```python
from build123d import *

# Parameters (mm, degrees)
F2_DEPTH  = 3
F1_R      = 2.5
F1_R_2    = 1.25
F3_DEPTH  = 10
F4_SIZE2  = 3
F4_SIZE   = 2
F5_R      = 2.99999
F7_W      = 10
F7_H      = 18
F8_DEPTH  = 4
F10_SIZE  = 1
F11_DEPTH = 33.6


# Not quite as in the source:
# - a fillet or chamfer is up to 0.001 mm smaller than in the source, because OpenCascade refuses the exact size


with BuildPart() as f2:
    # F0 (on Top) → F2 (new body)
    with BuildSketch(Plane.XY):
        with BuildLine():
            ThreePointArc((46, 18), (43.0710678119, 25.0710678119), (36, 28))
            Line((36, 28), (-36, 28))
            ThreePointArc((-36, 28), (-43.0710678119, 25.0710678119), (-46, 18))
            Line((-46, 18), (-46, -18))
            ThreePointArc((-46, -18), (-43.0710678119, -25.0710678119), (-36, -28))
            Line((-36, -28), (36, -28))
            ThreePointArc((36, -28), (43.0710678119, -25.0710678119), (46, -18))
            Line((46, -18), (46, 18))
        make_face()
    extrude(amount=F2_DEPTH)

    # F1 (on Top) → F3 (join)
    with BuildSketch(Plane.XY):
        with Locations((-29, 11.5)):
            Circle(F1_R)
        with Locations((-29, 11.5)):
            Circle(F1_R_2, mode=Mode.SUBTRACT)
        with Locations((29, 11.5)):
            Circle(F1_R)
        with Locations((29, 11.5)):
            Circle(F1_R_2, mode=Mode.SUBTRACT)
        with Locations((-29, -11.5)):
            Circle(F1_R)
        with Locations((-29, -11.5)):
            Circle(F1_R_2, mode=Mode.SUBTRACT)
        with Locations((29, -11.5)):
            Circle(F1_R)
        with Locations((29, -11.5)):
            Circle(F1_R_2, mode=Mode.SUBTRACT)
    extrude(amount=F3_DEPTH)

    # F4
    f4_edges = [f2.edges().sort_by_distance(p)[0] for p in [
        (-31.5, 11.5, 3),
        (26.5, 11.5, 3),
        (26.5, -11.5, 3),
        (-31.5, -11.5, 3),
    ]]
    chamfer(f4_edges, length=F4_SIZE, length2=F4_SIZE2)

    # F5 (radius 3 in the source; OpenCascade refuses exactly that, so slightly less here)
    f5_edges = [f2.edges().sort_by_distance(p)[0] for p in [
        (0, 28, 3),
    ]]
    fillet(f5_edges, radius=F5_R)

    # F7 (on offset) → F8 (join)
    with BuildSketch(Plane.YZ.offset(46)):
        with Locations((0, 9)):
            Rectangle(F7_W, F7_H)
    extrude(amount=-F8_DEPTH)

    # F9: F2 across plane


with BuildPart() as f2_1:
    add(f2.part)
    add(f2.part.mirror(Plane.YZ))

    # F10
    f10_edges = [f2_1.edges().sort_by_distance(p)[0] for p in [
        (-46, 0, 18),
        (46, 0, 18),
    ]]
    chamfer(f10_edges, length=F10_SIZE)

    # F11 (add): a face of the model
    f11_faces = [f2_1.faces().sort_by_distance(p)[0] for p in [
        (0, 0, 3),
    ]]
    extrude(f11_faces, amount=F11_DEPTH)


solid = f2_1.part
```
Here's how the part is built. I have some questions about the finished solid (model axes, mm). A direction names the side the tool comes from. Give positions to 0.01 mm unless a question says otherwise; leave off trailing zeros. Order: outer loops, then holes, each group sorted by start corner. A loop starts at its lowest first (then second) coordinate and runs counter-clockwise, first axis right, second up. Notation, with made-up numbers: M 36,1 L 74,1 A30 ccw 74,28 Z; hole C 14.5,67 d4. An arc over 180 degrees is marked long. Use a Markdown table: item, result. Add a question column.
1. For pin 1 Ø5 at (x, y) = (20.5, -5) entering from -Z; pin 2 Ø0.8 at (x, y) = (-29.5, 11) entering from +Z; pin 3 Ø0.9 at (x, z) = (-44.5, 8) entering from -Y; pin 4 Ø0.8 at (x, z) = (42.5, 29.5) entering from +Y, each with a flat end and sliding along its axis, tell me the tip position at first contact or that it passes through.
2. If we mould it in two halves opening along Y, with no side actions, what happens to faces 4 (the cylindrical face through (-24.708, 10.148, 19.565)), 5 (the flat face through (1, 0, 0)), 6 (the flat face through (-1, -25, 20)), 7 (the cylindrical face through (-0.5, 27.1, 2.14))? For each: +Y half, -Y half, draft (parallel to the pull), parting line (faces both ways), or undercut.
3. I need wall thicknesses on probe 1 along X at (y, z) = (-11.5, 27); probe 2 along Y at (x, z) = (29, 23); probe 3 along X at (y, z) = (-8.5, 30). Which ranges of each line are inside material? Lowest first, please. Write a range as from..to.
4. On a 3-axis mill with a long thin cutter (end or side, diameter ignored), from which of +Z, -Z, +X, -X, +Y, -Y can I reach the whole of each face in a straight line? I mean faces 1 (the flat face through (29, 12, 3)), 2 (the cylindrical face through (45.1, 11.59, 2.14)), 3 (the cylindrical face through (45.1, -11.41, 2.14)). Say none if no direction works.
5. Suppose I cut it at C-C (z = 15). List the corners of the cut face in (x, y) for me, and give its area (3 significant figures).
Results list:
| question | item | result |
|---|---|---|
| 1 | pin 1 | stops at z = 0 |
| 1 | pin 2 | stops at z = 3 |
| 1 | pin 3 | stops at y = -5 |
| 1 | pin 4 | stops at y = 21.43 |
| 2 | face 4 | undercut |
| 2 | face 5 | draft |
| 2 | face 6 | -Y half |
| 2 | face 7 | +Y half |
| 3 | probe 1 | x = -43..-33.5, -24.5..24.5, 33.5..43 |
| 3 | probe 2 | y = -25..-16, -7..7, 16..25 |
| 3 | probe 3 | x = -43..-32.35, -25.65..25.65, 32.35..43 |
| 4 | face 1 | +Z |
| 4 | face 2 | +Z, +X, +Y |
| 4 | face 3 | +Z, +X, -Y |
| 5 | outline | M -46,-5 L -43,-5 L -43,-18 A7 ccw -36,-25 L 36,-25 A7 ccw 43,-18 L 43,-5 L 46,-5 L 46,5 L 43,5 L 43,18 A7 ccw 36,25 L -36,25 A7 ccw -43,18 L -43,5 L -46,5 Z; hole C -29,-11.5 d9; hole C -29,11.5 d9; hole C 29,-11.5 d9; hole C 29,11.5 d9 |
| 5 | area | 4,060 mm² |
